Autodesk Inventor part; units mm, degrees
ref_plane "YZ Plane" through (0, 0, 0) normal (1, 0, 0) x (0, 1, 0)
ref_plane "XZ Plane" through (0, 0, 0) normal (0, 1, 0) x (-1, 0, 0)
ref_plane "XY Plane" through (0, 0, 0) normal (0, 0, 1) x (1, 0, 0)
sketch "Szkic8" plane through (0, 0, 0) normal (0, 1, 0) x (-1, 0, 0)
  circle A0 centre (0, 0) radius 50.8
  circle A1 centre (0, 0) radius 49.6
  dimension "d53" = 101.6
  dimension "d54" = 1.2
extrude "Wyciągnięcie proste2" add sketch "Szkic8" along normal mid plane 300
sketch "Szkic13" plane through (0, 0, 0) normal (0, 0, 1) x (1, 0, 0)
  circle A0 centre (0, 0) radius 12.5
  circle A1 centre (0, 0) radius 11.3
  dimension "d67" = 25
  dimension "d68" = 1.2
extrude "Wyciągnięcie proste6" add sketch "Szkic13" along normal blind 52
sketch "Szkic14" plane through (0, 0, 52) normal (0, 0, 1) x (1, 0, 0)
  circle A0 centre (0, 0) radius 11.3
extrude "Wyciągnięcie proste7" cut sketch "Szkic14" against normal blind 52
sketch "Szkic15" plane through (0, -150, 0) normal (0, -1, 0) x (1, 0, 0)
  circle A0 centre (0, 0) radius 49.6
extrude "Wyciągnięcie proste8" cut sketch "Szkic15" against normal blind 300
fillet "Zaokrąglenie3" radius 1.2 2 edges at (0, 12.5, 50.8) (-0.0026, -12.5, 50.8)
fillet "Zaokrąglenie4" radius 2.4 2 edges at (0.0388, -11.2999, 49.6) (-0.0376, 11.2999, 49.6)
equation "\"d53\" = OD"
equation "\"d54\" = THK"
equation "\"d55\" = L1"
equation "\"d67\" = OD2"
equation "\"d68\" = THK"
equation "\"d69\" = L2"
equation "\"d71\" = L2"
equation "\"d73\" = L1"
equation "\"d75\" = THK"
equation "\"d76\" = 2 * THK"
equation "\"SzerokośćGięciaPodcięcia\" = Grubość"
equation "\"RozmiarPodcięciaNarożnika\" = 4 * Grubość"
equation "\"PromieńPrzejścia\" = PromieńGięcia"
equation "\"Rozmiar_promienia_Jacobiego\" = PromieńGięcia"
equation "\"Wielk_odstępu\" = Grubość"
equation "\"d2\" = PromieńGięcia"
equation "\"d23\" = PromieńGięcia"
equation "\"OD\" = 101.6"
equation "\"THK\" = 1.2"
equation "\"L1\" = 300"
equation "\"L2\" = 52"
equation "\"OD2\" = 25"
properties part number "Trójnik red. krótki  Ø101,6 25 101,6 s=1,2 L=300" material "304"
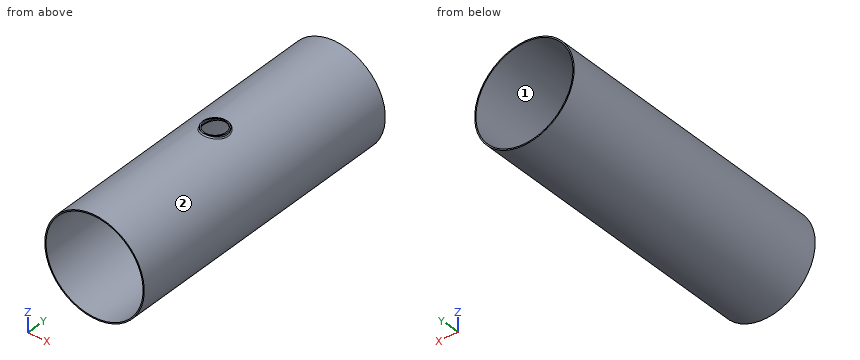
Design review of the part built by this model. Coordinates are the model's own, in mm. Face numbers are marked on the shaded views. Round coordinates to 2 decimals unless told otherwise and drop trailing zeros. Loops run counter-clockwise (first coordinate to the right, second up) from the corner with the lowest first, then second, coordinate; pieces in that order, holes last. Notation, with made-up numbers: (0, 75.25) -> (52, 75.25) arc R26 ccw to (52, 90.25) -> close; hole circle Ø1 at (88, 79). An arc over 180 degrees is marked (long way). Use one line per item in the form item = value. Start each with the question number.
Q1. We need section B-B on y = 42.5. Give the boundary of the cut face in (x, z), then the cut area to 4 significant figures.
Q2. We need section C-C on x = -17. Give the boundary of the cut face in (y, z).
Q3. For pin 1 Ø8 at (x, y) = (21, 12.5) entering from +Z; pin 2 Ø1.5 at (x, y) = (14, 5) entering from +Z; pin 3 Ø8 at (y, z) = (-43.5, 6.5) entering from +X, all flat-tipped, find the tip position at first contact; note any pin that passes through.
Q4. Wall thickness on line 1 along Z through (x, y) = (0, 72.5); line 2 along X through (y, z) = (0, 50); line 3 along X through (y, z) = (112, -16.5): over which ranges is each line inside the solid? List them lowest first. Write a range as [from, to].
Q5. We need section A-A on z = 10.5. Give the boundary of the cut face in (x, y), then the cut area to 3 significant figures.
Q6. Draft analysis for pull direction Z (two halves, no side actions). For the marked faces 1 and 2, state which applies: +Z half, -Z half, draft (parallel to the pull), parting line (faces both ways), or undercut.
Q7. We need section D-D on x = 4. State how many separate pieces and enclosed holes the cut face has, then the cut area to 3 significant figures.
Calculated:
q1.outline = circle Ø101.6 at (0, 0); hole circle Ø99.2 at (0, 0)
q1.area = 378.5 mm²
q2.outline = (-150, -47.87) -> (150, -47.87) -> (150, -46.6) -> (-150, -46.6) -> close; (-150, 46.6) -> (150, 46.6) -> (150, 47.87) -> (-150, 47.87) -> close
q3.pin_1 = 47.87
q3.pin_2 = 49.04
q3.pin_3 = 50.74
q4.line_1 = [-50.8, -49.6], [49.6, 50.8]
q4.line_2 = [-12.51, -11.31], [11.31, 12.51]
q4.line_3 = [-48.05, -46.78], [46.78, 48.05]
q5.outline = (-49.7, -150) -> (-48.48, -150) -> (-48.48, 150) -> (-49.7, 150) -> close; (48.48, -150) -> (49.7, -150) -> (49.7, 150) -> (48.48, 150) -> close
q5.area = 736 mm²
q6.face_1 = undercut
q6.face_2 = parting line
q7.separate_pieces = 3
q7.enclosed_holes = 0
q7.area = 698 mm²
